```python
from build123d import *

# Parameters (mm, degrees)
SKETCH_W        = 58
SKETCH_H        = 54
SKETCH_W_2      = 10
SKETCH_H_2      = 38
PAD_DEPTH       = 15
PAD001_DEPTH    = 40
SKETCH002_W     = 10
SKETCH002_H     = 38
SKETCH002_W_2   = 6
SKETCH002_H_2   = 33.513506
PAD002_DEPTH    = 10
SKETCH004_R     = 5
POCKET_DEPTH    = 5
SKETCH005_R     = 3
POCKET001_DEPTH = 10


with BuildPart() as part:
    # Sketch → Pad (new body)
    with BuildSketch(Plane.XY):
        with Locations((29, 27)):
            Rectangle(SKETCH_W, SKETCH_H)
        with Locations((31, 27)):
            Rectangle(SKETCH_W_2, SKETCH_H_2, mode=Mode.SUBTRACT)
    extrude(amount=PAD_DEPTH)

    # Sketch003 → Pad001 (new body)
    with BuildSketch(Plane.XY):
        Polygon((-15, 0), (-15, 14.5), (-10, 12), (-10, 42), (-15, 39.5), (-15, 54), (0, 54), (0, 0), align=None)
    extrude(amount=PAD001_DEPTH)

    # Sketch002 → Pad002 (new body)
    with BuildSketch(Plane.XY):
        with Locations((31, 27)):
            Rectangle(SKETCH002_W, SKETCH002_H)
        with Locations((31, 26.915923)):
            Rectangle(SKETCH002_W_2, SKETCH002_H_2, mode=Mode.SUBTRACT)
    extrude(amount=PAD002_DEPTH)

    # Sketch004 → Pocket (cut)
    with BuildSketch(Plane.YZ):
        with Locations((27, 27.5)):
            Circle(SKETCH004_R)
    extrude(amount=-POCKET_DEPTH, mode=Mode.SUBTRACT)

    # Sketch005 → Pocket001 (cut)
    with BuildSketch(Plane.YZ):
        with Locations((27, 27.5)):
            Circle(SKETCH005_R)
    extrude(amount=-POCKET001_DEPTH, mode=Mode.SUBTRACT)


solid = part.part
```
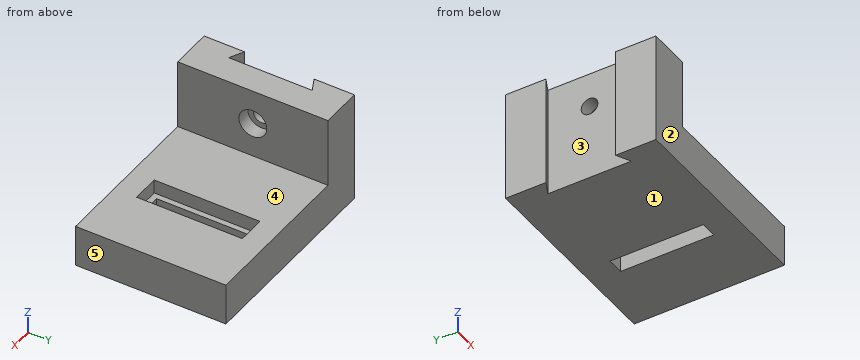
Part model, mm, in its own coordinate system. Face numbers are marked on the shaded views. A direction names the side the tool comes from. Coordinates: 2 decimals unless noted, no trailing zeros. Order: outer loops, then holes, each group sorted by start corner. A loop starts at its lowest first (then second) coordinate and runs counter-clockwise, first axis right, second up. Notation, with made-up numbers: (-7, 47) - (27, 47) arc R20 cw to (27, 73) - close; hole circle Ø3 at (-11, -31.5). An arc over 180 degrees is marked (long way). Return JSON: item names as keys, results as strings. Group by question number.
Item 1: Pull direction Y, two halves, no side cores. Call the marked faces 1, 2 and 3: pulls with the +Y half, pulls with the -Y half, needs draft (parallel to the pull), parting line crosses it, or undercut.
Item 2: Drill centre lines: probe 1 along Z at (x, y) = (-6.6, 27); probe 2 along X at (y, z) = (22, 12.5); probe 3 along Z at (x, y) = (-2.15, 27). Where is each one in solid material? Low to high. Write a range as from..to.
Item 3: Cut at A-A (z = 27.5). List the corners of the cut face in (x, y).
Item 4: Cut at B-B (y = 27). List the corners of the cut face in (x, z).
Item 5: Which spindle directions (+Z, -Z, +X, -X, +Y, -Y) get a long thin tool onto all of the face, cutting with end or side? Do the marked faces 4 and 5. Say none if no direction does.
Item 6: Cut at C-C (y = 35). List the corners of the cut face in (x, z), plus the area to 3 significant figures.
Item 7: Cut at D-D (z = 5.5). List the corners of the cut face in (x, y), plus the area to 3 significant figures.
Item 8: Pin check, flat tips, straight feed: pin 1 (6 mm diameter, centred on x = 4, y = 44.5, fed in from +Z); pin 2 (8 mm diameter, centred on y = 27, z = 27.5, fed in from -X); pin 3 (5 mm diameter, centred on y = 25.5, z = 27, fed in from +X). Stop position of each tip, or through.
Check values:
{
 "1": {"face 1": "needs draft", "face 2": "pulls with the -Y half", "face 3": "undercut"},
 "2": {"probe 1": "z = 0..24.5, 30.5..40", "probe 2": "x = -10..26, 36..58", "probe 3": "z = 0..22.5, 32.5..40"},
 "3": {"outline": "(-15, 0) - (0, 0) - (0, 22) - (-5, 22) - (-5, 24) - (-10, 24) - (-10, 12) - (-15, 14.5) - close; (-15, 39.5) - (-10, 42) - (-10, 30) - (-5, 30) - (-5, 32) - (0, 32) - (0, 54) - (-15, 54) - close"},
 "4": {"outline": "(-10, 0) - (28, 0) - (28, 10) - (26, 10) - (26, 15) - (0, 15) - (0, 22.5) - (-5, 22.5) - (-5, 24.5) - (-10, 24.5) - close; (-10, 30.5) - (-5, 30.5) - (-5, 32.5) - (0, 32.5) - (0, 40) - (-10, 40) - close; (34, 0) - (58, 0) - (58, 15) - (36, 15) - (36, 10) - (34, 10) - close"},
 "5": {"face 4": "+Z, +X, +Y, -Y", "face 5": "+Z, -Z, +X, +Y, -Y"},
 "6": {"outline": "(-10, 0) - (28, 0) - (28, 10) - (26, 10) - (26, 15) - (0, 15) - (0, 40) - (-10, 40) - close; (34, 0) - (58, 0) - (58, 15) - (36, 15) - (36, 10) - (34, 10) - close", "area": "1,160 mm2"},
 "7": {"outline": "(-15, 0) - (58, 0) - (58, 54) - (-15, 54) - (-15, 39.5) - (-10, 42) - (-10, 12) - (-15, 14.5) - close; hole (28, 10.16) - (34, 10.16) - (34, 43.67) - (28, 43.67) - close", "area": "3,600 mm2"},
 "8": {"pin 1": "stops at z = 15", "pin 2": "stops at x = -10", "pin 3": "stops at x = -5"}
}
